```python
from build123d import *

# Parameters (mm, degrees)
SKETCH1_R           = 30
SKETCH1_R_2         = 3
BOSS_EXTRUDE1_DEPTH = 10
SKETCH3_R           = 3
CUT_EXTRUDE1_DEPTH  = 44.588989435
CIRPATTERN1_COUNT   = 8
FILLET1_R           = 3


with BuildPart() as part:
    # Sketch1 → Boss-Extrude1 (new body)
    with BuildSketch(Plane(origin=(0, 0, 0), x_dir=(1, 0, 0), z_dir=(0, 1, 0))):
        with Locations(Location((0, 0, 0), (0, 0, 270))):
            Circle(SKETCH1_R)
        with Locations(Location((0, 25, 0), (0, 0, 270))):
            Circle(SKETCH1_R_2, mode=Mode.SUBTRACT)
        with Locations(Location((21.650635095, -12.5, 0), (0, 0, 270))):
            Circle(SKETCH1_R_2, mode=Mode.SUBTRACT)
        with Locations(Location((-21.650635095, -12.5, 0), (0, 0, 270))):
            Circle(SKETCH1_R_2, mode=Mode.SUBTRACT)
    extrude(amount=BOSS_EXTRUDE1_DEPTH)

    # Sketch3 → Cut-Extrude1 (cut, through all)
    with BuildSketch(Plane.XY):
        with Locations(Location((0, 5, 0), (0, 0, 90))):
            Circle(SKETCH3_R)
    cut_extrude1 = extrude(amount=CUT_EXTRUDE1_DEPTH, mode=Mode.SUBTRACT)

    # CirPattern1: Cut-Extrude1 ×8 about axis, 5 skipped
    cirpattern1_axis = Axis((0, 10, 0), (0, 1, 0))
    add([cut_extrude1.rotate(cirpattern1_axis, i * 360 / CIRPATTERN1_COUNT) for i in range(1, CIRPATTERN1_COUNT) if i not in (1, 2, 4, 6, 7)], mode=Mode.SUBTRACT)

    # Fillet1
    # the kernel refuses this fillet: 3 mm, written as the material it takes off along each edge
    with BuildSketch(Plane(origin=(0, 0, 0), x_dir=(0, 0, 1), z_dir=(-1, 0, 0))) as fillet1_piece_1:
        with BuildLine():
            CenterArc((30 - FILLET1_R, FILLET1_R), FILLET1_R, 270, 90)
            Line((30 - FILLET1_R, 0), (30, 0))
            Line((30, 0), (30, FILLET1_R))
        make_face()
    revolve(axis=Axis((0, 0, 0), (0, 1, 0)), mode=Mode.SUBTRACT)
    with BuildSketch(Plane(origin=(0, 10, 0), x_dir=(0, 0, 1), z_dir=(-1, 0, 0))) as fillet1_piece_2:
        with BuildLine():
            CenterArc((30 - FILLET1_R, -FILLET1_R), FILLET1_R, 0, 90)
            Line((30 - FILLET1_R, 0), (30, 0))
            Line((30, 0), (30, -FILLET1_R))
        make_face()
    revolve(axis=Axis((0, 10, 0), (0, 1, 0)), mode=Mode.SUBTRACT)


solid = part.part
```
For this review, take the finished solid that the model builds, in its own axes (mm). Coordinates: 2 decimals unless noted, no trailing zeros. Write each loop counter-clockwise with the first axis right and the second up, starting at its lowest first coordinate (ties: lowest second). Pieces come first, ordered by that corner, then holes.
(1) For pin 1 Ø2 at (y, z) = (2, 23.5) entering from -X; pin 2 Ø6 at (x, y) = (-21, 6) entering from -Z, all flat-tipped, find the tip position at first contact; note any pin that passes through.
(2) Add section D-D on y = 1. Give the boundary of the cut face in (x, z), then the cut area to 3 significant figures.
(3) The part is to be moulded in two halves that separate along Y. For faces 1 (the face through (0, 0, 0)), 2 (the face through (0, 5, -28)), 3 (the face through (0, 2, 15)), say which applies: +Y half, -Y half, draft (parallel to the pull), parting line (faces both ways), or undercut.
(4) Add section B-B on z = 12.5. Count the separate pieces of the cut face and the enclosed holes in it, then the cut area to 3 significant figures.
(5) Add section A-A on y = 6.25. Give the boundary of the cut face in (x, z).
(6) Wall thickness on probe 1 along Y at (x, z) = (0, 11.5); probe 2 along X at (y, z) = (4, 10); probe 3 along X at (y, z) = (2.5, 11): over which ranges is each line inside the solid? List them lowest first.
Answer sheet:
1. pin 1: stops at x = -19.67
1. pin 2: stops at z = -24
2. outline: circle Ø58.47 at (0, 0); hole circle Ø6 at (-21.65, 12.5); hole circle Ø6 at (0, -25); hole circle Ø6 at (21.65, 12.5)
2. area: 2,600 mm2
3. face 1: -Y half
3. face 2: draft
3. face 3: undercut
4. separate pieces: 3
4. enclosed holes: 1
4. area: 389 mm2
5. outline: (-23.05, -19.2) - (-2.73, 1.13) - (-2.73, 29.88) arc R30 ccw to start; (-19.2, -23.05) arc R30 ccw to (19.2, -23.05) - (0, -3.86) - close; (2.73, 1.13) - (23.05, -19.2) arc R30 ccw to (2.73, 29.88) - close; hole circle Ø6 at (-21.65, 12.5); hole circle Ø6 at (0, -25); hole circle Ø6 at (21.65, 12.5)
6. probe 1: y = 0 to 2, 8 to 10
6. probe 2: x = -28.28 to -23.31, -19.99 to -2.83, 2.83 to 19.99, 23.31 to 28.28
6. probe 3: x = -27.87 to -24.25, -19.05 to -1.66, 1.66 to 19.05, 24.25 to 27.87
